from build123d import *

# Parameters (mm, degrees)
SKETCH1_W             = 45
SKETCH1_H             = 36.5
BOSS_EXTRUDE1_DEPTH   = 10
SKETCH1_R             = 36.5
SKETCH1_R_2           = 2.25
SKETCH1_W_2           = 55
SKETCH1_H_2           = 46.5
BOSS_EXTRUDE1_2_DEPTH = 10
SKETCH1_2_W           = 55
SKETCH1_2_H           = 46.5
SKETCH1_2_W_2         = 45
SKETCH1_2_H_2         = 36.5
BOSS_EXTRUDE2_DEPTH   = 60
FILLET2_R             = 1
CUT_EXTRUDE1_START    = -5
SKETCH2_W             = 36.5
SKETCH2_H             = 50
CUT_EXTRUDE1_DEPTH    = 6
BOSS_EXTRUDE3_START   = -5
SKETCH3_W             = 46.5
SKETCH3_H             = 13.75
BOSS_EXTRUDE3_DEPTH   = 5
FILLET5_R             = 2.5
SKETCH6_R             = 4.4
CUT_EXTRUDE4_DEPTH    = 6
SKETCH7_R             = 19
SKETCH7_R_2           = 14
BOSS_EXTRUDE4_DEPTH   = 5.5
SKETCH7_2_R           = 14
CUT_EXTRUDE5_DEPTH    = 3
SKETCH8_R             = 1.25
CUT_EXTRUDE6_DEPTH    = 11
SKETCH9_R             = 1.25
CUT_EXTRUDE7_DEPTH    = 1
SKETCH11_W            = 45
SKETCH11_H            = 36.5
BOSS_EXTRUDE5_DEPTH   = 15
SKETCH12_W            = 5
SKETCH12_H            = 36.5
BOSS_EXTRUDE6_DEPTH   = 15
BOSS_EXTRUDE7_START   = 15
SKETCH13_R            = 1.25
BOSS_EXTRUDE7_DEPTH   = 15
CUT_EXTRUDE8_DEPTH    = 3
SKETCH15_W            = 20
SKETCH15_H            = 20
CUT_EXTRUDE9_DEPTH    = 114.850371766


with BuildPart() as part:
    # Sketch1 → Boss-Extrude1 (new body)
    with BuildSketch(Plane(origin=(0, 0, 0), x_dir=(1, 0, 0), z_dir=(0, 1, 0))):
        Rectangle(SKETCH1_W, SKETCH1_H)
    extrude(amount=BOSS_EXTRUDE1_DEPTH)



with BuildPart() as body_2:
    # Sketch1 → Boss-Extrude1 2 (new body)
    with BuildSketch(Plane(origin=(0, 0, 0), x_dir=(1, 0, 0), z_dir=(0, 1, 0))):
        with Locations(Location((0, 0, 0), (0, 0, 270))):
            Circle(SKETCH1_R)
        with Locations(Location((-15.89, -27.522287332, 0), (0, 0, 270))):
            Circle(SKETCH1_R_2, mode=Mode.SUBTRACT)
        with Locations(Location((15.89, -27.522287332, 0), (0, 0, 270))):
            Circle(SKETCH1_R_2, mode=Mode.SUBTRACT)
        with Locations(Location((-31.78, 0, 0), (0, 0, 270))):
            Circle(SKETCH1_R_2, mode=Mode.SUBTRACT)
        with Locations(Location((-15.89, 27.522287332, 0), (0, 0, 270))):
            Circle(SKETCH1_R_2, mode=Mode.SUBTRACT)
        Rectangle(SKETCH1_W_2, SKETCH1_H_2, mode=Mode.SUBTRACT)
        with Locations(Location((31.78, 0, 0), (0, 0, 270))):
            Circle(SKETCH1_R_2, mode=Mode.SUBTRACT)
        with Locations(Location((15.89, 27.522287332, 0), (0, 0, 270))):
            Circle(SKETCH1_R_2, mode=Mode.SUBTRACT)
    extrude(amount=BOSS_EXTRUDE1_2_DEPTH)

    # Sketch1<2> → Boss-Extrude2 (add)
    with BuildSketch(Plane(origin=(0, 0, 0), x_dir=(1, 0, 0), z_dir=(0, 1, 0))):
        Rectangle(SKETCH1_2_W, SKETCH1_2_H)
        Rectangle(SKETCH1_2_W_2, SKETCH1_2_H_2, mode=Mode.SUBTRACT)
    extrude(amount=BOSS_EXTRUDE2_DEPTH)

    # Fillet2
    fillet2_edges = [body_2.edges().sort_by_distance(p)[0] for p in [
        (-22.5, 30, -18.25),
        (22.5, 30, -18.25),
        (22.5, 30, 18.25),
        (-22.5, 30, 18.25),
    ]]
    fillet(fillet2_edges, radius=FILLET2_R)

    # Sketch2 → Cut-Extrude1 (cut)
    with BuildSketch(Plane(origin=(-22.5, 0, 0), x_dir=(0, 0, -1), z_dir=(1, 0, 0)).offset(CUT_EXTRUDE1_START)):
        with Locations((0, 35)):
            Rectangle(SKETCH2_W, SKETCH2_H)
    extrude(amount=CUT_EXTRUDE1_DEPTH, mode=Mode.SUBTRACT)

    # Sketch3 → Boss-Extrude3 (add)
    with BuildSketch(Plane.ZY.offset(27.5).offset(BOSS_EXTRUDE3_START)):
        with Locations((0, 16.875)):
            Rectangle(SKETCH3_W, SKETCH3_H)
    extrude(amount=BOSS_EXTRUDE3_DEPTH)

    # Fillet5
    fillet5_edges = [body_2.edges().sort_by_distance(p)[0] for p in [
        (27.5, 35, -23.25),
        (-27.5, 35, -23.25),
        (-27.5, 35, 23.25),
        (27.5, 35, 23.25),
    ]]
    fillet(fillet5_edges, radius=FILLET5_R)

    # Sketch6 → Cut-Extrude4 (cut)
    with BuildSketch(Plane(origin=(0, 10, 0), x_dir=(1, 0, 0), z_dir=(0, 1, 0))):
        with Locations(Location((-15.89, 27.522287332, 0), (0, 0, 270))):
            Circle(SKETCH6_R)
        with Locations(Location((15.89, 27.522287332, 0), (0, 0, 270))):
            Circle(SKETCH6_R)
        with Locations(Location((31.78, 0, 0), (0, 0, 270))):
            Circle(SKETCH6_R)
        with Locations(Location((15.89, -27.522287332, 0), (0, 0, 270))):
            Circle(SKETCH6_R)
        with Locations(Location((-15.89, -27.522287332, 0), (0, 0, 270))):
            Circle(SKETCH6_R)
        with Locations(Location((-31.78, 0, 0), (0, 0, 270))):
            Circle(SKETCH6_R)
    extrude(amount=-CUT_EXTRUDE4_DEPTH, mode=Mode.SUBTRACT)

    # Sketch7 → Boss-Extrude4 (add)
    with BuildSketch(Plane(origin=(27.5, 0, 0), x_dir=(0, 0, -1), z_dir=(1, 0, 0))):
        with Locations(Location((0, 52.25, 0), (0, 0, 155.927346102))):
            Circle(SKETCH7_R)
        with Locations(Location((0, 52.25, 0), (0, 0, 146.387625402))):
            Circle(SKETCH7_R_2, mode=Mode.SUBTRACT)
    extrude(amount=BOSS_EXTRUDE4_DEPTH)

    # Sketch7<2> → Cut-Extrude5 (cut)
    with BuildSketch(Plane(origin=(27.5, 0, 0), x_dir=(0, 0, -1), z_dir=(1, 0, 0))):
        with Locations(Location((0, 52.25, 0), (0, 0, 146.387625402))):
            Circle(SKETCH7_2_R)
    extrude(amount=-CUT_EXTRUDE5_DEPTH, mode=Mode.SUBTRACT)

    # Sketch8 → Cut-Extrude6 (cut)
    with BuildSketch(Plane(origin=(0, 60, 0), x_dir=(1, 0, 0), z_dir=(0, 1, 0))):
        with Locations(Location((-25, 20.75, 0), (0, 0, 270))):
            Circle(SKETCH8_R)
        with Locations(Location((25, 20.75, 0), (0, 0, 270))):
            Circle(SKETCH8_R)
        with Locations(Location((25, -20.75, 0), (0, 0, 270))):
            Circle(SKETCH8_R)
        with Locations(Location((-25, -20.75, 0), (0, 0, 270))):
            Circle(SKETCH8_R)
    extrude(amount=-CUT_EXTRUDE6_DEPTH, mode=Mode.SUBTRACT)

    # Sketch9 → Cut-Extrude7 (cut)
    with BuildSketch(Plane(origin=(0, 60, 0), x_dir=(1, 0, 0), z_dir=(0, 1, 0))):
        with BuildLine():
            Line((21.5, -18.25), (-27.5, -18.25))
            Line((-27.5, -18.25), (-27.5, -20.75))
            ThreePointArc((-27.5, -20.75), (-26.767766953, -22.517766953), (-25, -23.25))
            Line((-25, -23.25), (25, -23.25))
            ThreePointArc((25, -23.25), (26.767766953, -22.517766953), (27.5, -20.75))
            Line((27.5, -20.75), (27.5, -17.347550259))
            Line((27.5, -17.347550259), (27.5, -11.659223816))
            Line((27.5, -11.659223816), (24.5, -11.659223816))
            Line((24.5, -11.659223816), (24.5, 11.659223816))
            Line((24.5, 11.659223816), (27.5, 11.659223816))
            Line((27.5, 11.659223816), (27.5, 17.347550259))
            Line((27.5, 17.347550259), (27.5, 20.75))
            ThreePointArc((27.5, 20.75), (26.767766953, 22.517766953), (25, 23.25))
            Line((25, 23.25), (-25, 23.25))
            ThreePointArc((-25, 23.25), (-26.767766953, 22.517766953), (-27.5, 20.75))
            Line((-27.5, 20.75), (-27.5, 18.25))
            Line((-27.5, 18.25), (21.5, 18.25))
            ThreePointArc((21.5, 18.25), (22.207106781, 17.957106781), (22.5, 17.25))
            Line((22.5, 17.25), (22.5, -17.25))
            ThreePointArc((22.5, -17.25), (22.207106781, -17.957106781), (21.5, -18.25))
        make_face()
        with Locations(Location((-25, -20.75, 0), (0, 0, 270))):
            Circle(SKETCH9_R, mode=Mode.SUBTRACT)
        with Locations(Location((25, -20.75, 0), (0, 0, 270))):
            Circle(SKETCH9_R, mode=Mode.SUBTRACT)
        with Locations(Location((25, 20.75, 0), (0, 0, 270))):
            Circle(SKETCH9_R, mode=Mode.SUBTRACT)
        with Locations(Location((-25, 20.75, 0), (0, 0, 270))):
            Circle(SKETCH9_R, mode=Mode.SUBTRACT)
    extrude(amount=-CUT_EXTRUDE7_DEPTH, mode=Mode.SUBTRACT)


with BuildPart() as part_1:
    add(part.part)

    add(body_2.part)  # Boss-Extrude5 merges body 2
    # Sketch11 → Boss-Extrude5 (add)
    with BuildSketch(Plane(origin=(0, 10, 0), x_dir=(1, 0, 0), z_dir=(0, 1, 0))):
        Rectangle(SKETCH11_W, SKETCH11_H)
    extrude(amount=BOSS_EXTRUDE5_DEPTH)

    # Sketch12 → Boss-Extrude6 (add)
    with BuildSketch(Plane(origin=(0, 23.75, 0), x_dir=(1, 0, 0), z_dir=(0, 1, 0))):
        with Locations((-25, 0)):
            Rectangle(SKETCH12_W, SKETCH12_H)
    extrude(amount=BOSS_EXTRUDE6_DEPTH)

    # Sketch13 → Boss-Extrude7 (add)
    with BuildSketch(Plane(origin=(0, 59, 0), x_dir=(1, 0, 0), z_dir=(0, 1, 0)).offset(BOSS_EXTRUDE7_START)):
        with BuildLine():
            Line((27.5, 12.265296572), (27.5, -12.265296572))
            Line((27.5, -12.265296572), (27.5, -17.760560239))
            Line((27.5, -17.760560239), (27.5, -20.75))
            ThreePointArc((27.5, -20.75), (26.767766953, -22.517766953), (25, -23.25))
            Line((25, -23.25), (-25, -23.25))
            ThreePointArc((-25, -23.25), (-26.767766953, -22.517766953), (-27.5, -20.75))
            Line((-27.5, -20.75), (-27.5, -18.25))
            Line((-27.5, -18.25), (21.5, -18.25))
            ThreePointArc((21.5, -18.25), (22.207106781, -17.957106781), (22.5, -17.25))
            Line((22.5, -17.25), (22.5, 17.25))
            ThreePointArc((22.5, 17.25), (22.207106781, 17.957106781), (21.5, 18.25))
            Line((21.5, 18.25), (-27.5, 18.25))
            Line((-27.5, 18.25), (-27.5, 20.75))
            ThreePointArc((-27.5, 20.75), (-26.767766953, 22.517766953), (-25, 23.25))
            Line((-25, 23.25), (25, 23.25))
            ThreePointArc((25, 23.25), (26.767766953, 22.517766953), (27.5, 20.75))
            Line((27.5, 20.75), (27.5, 17.760560239))
            Line((27.5, 17.760560239), (27.5, 12.265296572))
        make_face()
        with Locations(Location((-25, -20.75, 0), (0, 0, 270))):
            Circle(SKETCH13_R, mode=Mode.SUBTRACT)
        with Locations(Location((25, -20.75, 0), (0, 0, 270))):
            Circle(SKETCH13_R, mode=Mode.SUBTRACT)
        with Locations(Location((25, 20.75, 0), (0, 0, 270))):
            Circle(SKETCH13_R, mode=Mode.SUBTRACT)
        with Locations(Location((-25, 20.75, 0), (0, 0, 270))):
            Circle(SKETCH13_R, mode=Mode.SUBTRACT)
    extrude(amount=-BOSS_EXTRUDE7_DEPTH)

    # Sketch14 → Cut-Extrude8 (cut)
    with BuildSketch(Plane(origin=(27.5, 0, 0), x_dir=(0, 0, -1), z_dir=(1, 0, 0))):
        with BuildLine():
            Line((-12.265296572, 59), (12.265296572, 59))
            ThreePointArc((12.265296572, 59), (0, 66.25), (-12.265296572, 59))
        make_face()
    extrude(amount=-CUT_EXTRUDE8_DEPTH, mode=Mode.SUBTRACT)

    # Sketch15 → Cut-Extrude9 (cut, through all)
    with BuildSketch(Plane(origin=(26.767766953, 74, -22.517766953), x_dir=(-0.7071067811865468, 0, -0.7071067811865483), z_dir=(0.7071067811865483, 0, -0.7071067811865468))):
        with Locations((0, -51)):
            Rectangle(SKETCH15_W, SKETCH15_H)
    cut_extrude9 = extrude(amount=-CUT_EXTRUDE9_DEPTH, mode=Mode.SUBTRACT)

    # Mirror1: Cut-Extrude9 across plane
    add(cut_extrude9.mirror(Plane.XY), mode=Mode.SUBTRACT)


solid = part_1.part
Input: part model. Units: mm. Frame: model coordinates. A direction names the side the tool comes from. Coordinates: 2 decimals unless noted, no trailing zeros. Loops run counter-clockwise (first coordinate to the right, second up) from the corner with the lowest first, then second, coordinate; pieces in that order, holes last.
Q1. Cut plane B-B (x = 31.78). Output: boundary loops of the cut face in (y, z).
Q2. Material intervals for line 1 (Y direction, x = 28, z = 0); line 2 (Z direction, x = -3, y = 68); line 3 (Z direction, x = -15.89, y = 7.95), sorted ascending.
Q3. Cut plane A-A (y = 17). Output: boundary loops of the cut face in (x, z).
Q4. Contact query for flat-ended pins moving along their axis: pin 1 (8 mm diameter, centred on x = 15.89, z = -27.52, fed in from +Y); pin 2 (5 mm diameter, centred on y = 60.5, z = -15, fed in from -X); pin 3 (1.2 mm diameter, centred on x = 4, z = -17, fed in from +Y). Output: stop coordinate, or through.
Q5. Cut plane C-C (y = 52.25). Output: boundary loops of the cut face in (x, z).
Q6. Cut plane D-D (x = 15.89). Give the number of separate pieces and of enclosed holes in the cut face, then the cut area to 3 significant figures.
Q7. Set-up query: faces 1 (the face through (26.787, 11.521, 22.498)), 2 (the face through (-26.748, 11.521, 22.537)), 3 (the face through (-20.53, 20.64, 10.64)), 4 (the face through (-27.5, 28, 5)). Return all of +Z, -Z, +X, -X, +Y, -Y with unobstructed straight access to the full face (end or side cutting, diameter ignored); none if empty.
Q8. Draft query along Y for faces 5 (the face through (26.787, 53.787, 22.498)), 6 (the face through (4, 13, 0)), 7 (the face through (23, 74, 2)). Return one class per face: +Y half, -Y half, draft (parallel to the pull), parting line (faces both ways), or undercut.
Working result:
1. outline: (0, -17.95) - (10, -17.95) - (10, -4.4) - (4, -4.4) - (4, -2.25) - (0, -2.25) - close; (0, 2.25) - (4, 2.25) - (4, 4.4) - (10, 4.4) - (10, 17.95) - (0, 17.95) - close; circle Ø38 at (52.25, 0); hole circle Ø28 at (52.25, 0)
2. line 1: y = 0 to 4, 33.25 to 38.25, 66.25 to 71.25
2. line 2: z = -23.25 to -18.25, 18.25 to 23.25
2. line 3: z = -32.86 to -31.92, -23.12 to 23.12, 31.92 to 32.86
3. outline: (-27.5, -17.61) - (-9.89, 0) - (-27.5, 17.61) - close; (-4.86, -23.25) - (13.36, -23.25) - (4.25, -14.14) - close; (-4.86, 23.25) - (4.25, 14.14) - (13.36, 23.25) - close; (18.39, 0) - (27.5, -9.11) - (27.5, 9.11) - close
4. pin 1: stops at y = 4
4. pin 2: stops at x = 22.47
4. pin 3: stops at y = 25
5. outline: (-27.5, -20.75) arc R2.5 ccw to (-25, -23.25) - (25, -23.25) arc R2.5 ccw to (27.5, -20.75) - (27.5, -19) - (33, -19) - (33, -14) - (24.5, -14) - (24.5, 14) - (33, 14) - (33, 19) - (27.5, 19) - (27.5, 20.75) arc R2.5 ccw to (25, 23.25) - (-25, 23.25) arc R2.5 ccw to (-27.5, 20.75) - (-27.5, 18.25) - (21.5, 18.25) arc R1 cw to (22.5, 17.25) - (22.5, -17.25) arc R1 cw to (21.5, -18.25) - (-27.5, -18.25) - close; hole circle Ø2.5 at (-25, -20.75); hole circle Ø2.5 at (-25, 20.75); hole circle Ø2.5 at (25, -20.75); hole circle Ø2.5 at (25, 20.75)
6. separate pieces: 5
6. enclosed holes: 0
6. area: 1,070 mm2
7. face 1: +Z, +X, +Y
7. face 2: +Z, -X, +Y
7. face 3: +Z
7. face 4: +Z, -Z, -X, +Y
8. face 5: draft
8. face 6: undercut
8. face 7: +Y half
